Verification items for the finished model (mm, model axes). A direction names the side the tool comes from. Give positions to 0.01 mm unless a question says otherwise; leave off trailing zeros. Order: outer loops, then holes, each group sorted by start corner. A loop starts at its lowest first (then second) coordinate and runs counter-clockwise, first axis right, second up. Notation, with made-up numbers: (6, -33.75) - (57, -33.75) arc R21 cw to (57, -16.75) - close; hole circle Ø3 at (-33.5, 58.5). An arc over 180 degrees is marked (long way). Answer as a JSON object with one key per item and string values.
```python
from build123d import *

# Parameters (mm, degrees)
BOSS_EXTRUDE1_DEPTH             = 23
FILLET2_R                       = 50.8
SKETCH2_R                       = 40.05
CUT_EXTRUDE1_DEPTH              = 16
SKETCH5_R                       = 36.83
CUT_EXTRUDE2_DEPTH              = 25.4
FILLET5_R                       = 1
FILLET6_R                       = 1
CBORE_FOR_M10_SHCS7_D           = 10.5
CBORE_FOR_M10_SHCS7_CBORE_D     = 18
CBORE_FOR_M10_SHCS7_CBORE_DEPTH = 12
TAP_DRILL_FOR_M8X1_25_TAP2_D    = 6.8
F_8_0MM_DOWEL_HOLE1_D           = 8
F_8_0MM_DOWEL_HOLE1_DEPTH       = 9
F_8_0MM_DOWEL_HOLE1_TIP         = 2.403442476
F_10_0MM_DOWEL_HOLE3_D          = 10
F_10_0MM_DOWEL_HOLE3_DEPTH      = 10
F_10_0MM_DOWEL_HOLE3_TIP        = 3.004303095
CBORE_FOR_M10_SHCS9_D           = 10.5
CBORE_FOR_M10_SHCS9_CBORE_D     = 18
CBORE_FOR_M10_SHCS9_CBORE_DEPTH = 10


with BuildPart() as part:
    # Sketch1 → Boss-Extrude1 (new body)
    with BuildSketch(Plane.XY):
        with BuildLine():
            Line((84.221105008, -163.490124242), (2.699306526, -136.831626991))
            Line((2.699306526, -136.831626991), (-67.458438584, -162.730244564))
            ThreePointArc((-67.458438584, -162.730244564), (-75.680634631, -163.297391653), (-82.910842941, -159.341351783))
            Line((-82.910842941, -159.341351783), (-126.914053579, -115.336397895))
            ThreePointArc((-126.914053579, -115.336397895), (-130.093640928, -110.577690662), (-131.210211433, -104.964461595))
            Line((-131.210211433, -104.964461595), (-131.213297338, 125.035476514))
            ThreePointArc((-131.213297338, 125.035476514), (-126.350161673, 135.869915187), (-115.02264263, 139.436771249))
            Line((-115.02264263, 139.436771249), (-20.796830867, 128.37488637))
            Line((-20.796830867, 128.37488637), (49.24312976, 147.55277548))
            ThreePointArc((49.24312976, 147.55277548), (58.421803723, 147.044752766), (65.450410839, 141.119820294))
            Line((65.450410839, 141.119820294), (107.841002341, 71.642808501))
            ThreePointArc((107.841002341, 71.642808501), (117.701476238, 53.952608996), (124.683759391, 34.941564155))
            Line((124.683759391, 34.941564155), (145.845410308, -40.455794779))
            ThreePointArc((145.845410308, -40.455794779), (145.61886709, -49.11646402), (140.544799405, -56.138739339))
            Line((140.544799405, -56.138739339), (109.149264581, -79.773969292))
            Line((109.149264581, -79.773969292), (103.401152517, -150.732337669))
            ThreePointArc((103.401152517, -150.732337669), (96.90432541, -161.761540655), (84.221105008, -163.490124242))
        make_face()
    extrude(amount=BOSS_EXTRUDE1_DEPTH)

    # Fillet2
    fillet2_edges = [part.edges().sort_by_distance(p)[0] for p in [
        (109.149264581, -79.773969292, 11.5),
        (2.699306526, -136.831626991, 11.5),
        (-20.796830867, 128.37488637, 11.5),
    ]]
    fillet(fillet2_edges, radius=FILLET2_R)

    # Sketch2 → Cut-Extrude1 (cut)
    with BuildSketch(Plane(origin=(0, 0, 23), x_dir=(-1, 0, 0), z_dir=(0, 0, -1))):
        Circle(SKETCH2_R)
    extrude(amount=CUT_EXTRUDE1_DEPTH, mode=Mode.SUBTRACT)

    # Sketch5 → Cut-Extrude2 (cut)
    with BuildSketch(Plane(origin=(0, 0, 23), x_dir=(-1, 0, 0), z_dir=(0, 0, -1))):
        with Locations(Location((0, 0, 0), (0, 0, 180))):
            Circle(SKETCH5_R)
    extrude(amount=CUT_EXTRUDE2_DEPTH, mode=Mode.SUBTRACT)

    # Fillet5
    fillet5_edges = [part.edges().sort_by_distance(p)[0] for p in [
        (40.05, 0, 23),
    ]]
    fillet(fillet5_edges, radius=FILLET5_R)

    # Fillet6
    fillet6_edges = [part.edges().sort_by_distance(p)[0] for p in [
        (40.05, 0, 7),
    ]]
    fillet(fillet6_edges, radius=FILLET6_R)

    # CBORE for M10 SHCS7 (through all)
    with Locations(Plane.XY.offset(23)):
        with Locations((-116.713297339, 125.03567106), (-116.541509562, -104.964264785), (-72.538298924, -148.969218673)):
            CounterBoreHole(CBORE_FOR_M10_SHCS7_D / 2, CBORE_FOR_M10_SHCS7_CBORE_D / 2, CBORE_FOR_M10_SHCS7_CBORE_DEPTH)

    # Tap Drill for M8x1.25 Tap2 (through all)
    with Locations(Plane.XY.offset(23)):
        with Locations((46, 97.92), (-31, 98), (-105.616623552, 111.626092354), (-105.616623552, -112.292869781), (-31.12, -98.35), (45.85, -98.52), (78.925, -30.46), (77.9, 39.75)):
            Hole(TAP_DRILL_FOR_M8X1_25_TAP2_D / 2)

    # Ø8.0mm Dowel Hole1
    with Locations(Plane.XY.offset(23)):
        with Locations((-72, 97.977867106), (-72, -98.122132894)):
            Hole(F_8_0MM_DOWEL_HOLE1_D / 2, depth=F_8_0MM_DOWEL_HOLE1_DEPTH)
            with Locations((0, 0, -(F_8_0MM_DOWEL_HOLE1_DEPTH + F_8_0MM_DOWEL_HOLE1_TIP / 2))):  # 118° drill point
                Cone(0, F_8_0MM_DOWEL_HOLE1_D / 2, F_8_0MM_DOWEL_HOLE1_TIP, mode=Mode.SUBTRACT)

    # Ø10.0mm Dowel Hole3
    with Locations(Plane(origin=(0, 0, 0), x_dir=(-1, 0, 0), z_dir=(0, 0, -1))):
        with Locations((76.55340813, 103.753913834), (-59.102558089, -114.980445858)):
            Hole(F_10_0MM_DOWEL_HOLE3_D / 2, depth=F_10_0MM_DOWEL_HOLE3_DEPTH)
            with Locations((0, 0, -(F_10_0MM_DOWEL_HOLE3_DEPTH + F_10_0MM_DOWEL_HOLE3_TIP / 2))):  # 118° drill point
                Cone(0, F_10_0MM_DOWEL_HOLE3_D / 2, F_10_0MM_DOWEL_HOLE3_TIP, mode=Mode.SUBTRACT)

    # CBORE for M10 SHCS9 (through all)
    with Locations(Plane.XY.offset(23)):
        with Locations((53.072470058, 133.567563544), (131.722431635, -44.419667636), (88.780343848, -149.547952394)):
            CounterBoreHole(CBORE_FOR_M10_SHCS9_D / 2, CBORE_FOR_M10_SHCS9_CBORE_D / 2, CBORE_FOR_M10_SHCS9_CBORE_DEPTH)


solid = part.part
```
(1) Section check A-A (x = 0). Record the cut outline in (y, z), then the cut area to 3 significant figures.
Computed values:
{"outline": "(-139.94, 0) - (-36.83, 0) - (-36.83, 7) - (-39.05, 7) arc R1 cw to (-40.05, 8) - (-40.05, 22) arc R1 ccw to (-41.05, 23) - (-139.94, 23) - close; (36.83, 0) - (134.07, 0) - (134.07, 23) - (41.05, 23) arc R1 ccw to (40.05, 22) - (40.05, 8) arc R1 cw to (39.05, 7) - (36.83, 7) - close", "area": "4,510 mm²"}
(2) Gauge pin test, flat ends, axial feed: pin 1 Ø9 at (x, y) = (53.5, 133.5) entering from +Z; pin 2 Ø13.5 at (x, y) = (-116.54, -104.96) entering from +Z; pin 3 Ø12 at (x, z) = (72.5, 7) entering from +Y; pin 4 Ø8 at (x, z) = (40, 16.5) entering from +Y. Record the tip position at first contact, or that the pin passes through.
Computed values:
{"pin 1": "passes through", "pin 2": "stops at z = 11", "pin 3": "stops at y = 139.4", "pin 4": "stops at y = 146.12"}
(3) Material ranges on line 1 along X through (y, z) = (-98, 8.5); line 2 along Y through (x, z) = (-33, 11.75); line 3 along Y through (x, z) = (-72, 19.5), recorded low to high. Write a range as [from, to].
Computed values:
{"line 1": "x = [-131.21, -34.5], [-27.74, 42.49], [49.21, 107.88]", "line 2": "y = [-150.01, -101.18], [-95.52, -22.69], [22.69, 95.25], [100.75, 129.81]", "line 3": "y = [-163.63, -157.95], [-139.99, -102.12], [-94.12, 93.98], [101.98, 134.39]"}
(4) Section check B-B (y = 0). Record the cut outline in (x, z), then the cut area to 3 significant figures.
Computed values:
{"outline": "(-131.21, 0) - (-36.83, 0) - (-36.83, 7) - (-39.05, 7) arc R1 cw to (-40.05, 8) - (-40.05, 22) arc R1 ccw to (-41.05, 23) - (-131.21, 23) - close; (36.83, 0) - (134.49, 0) - (134.49, 23) - (41.05, 23) arc R1 ccw to (40.05, 22) - (40.05, 8) arc R1 cw to (39.05, 7) - (36.83, 7) - close", "area": "4,310 mm²"}
(5) Section check D-D (y = -129.5). Record the cut outline in (x, z).
Computed values:
{"outline": "(-112.75, 0) - (105.12, 0) - (105.12, 23) - (-112.75, 23) - close"}
(6) Access from +Z, -Z, +X, -X, +Y, -Y to the whole of each face (thin tool, end or side, straight path). Record for faces 5 (the flat face through (-40.295, -152.703, 11.339)), 6 (the flat face through (105.38, -126.29, 11.34)), 7 (the flat face through (-112.7, -108.8, 11)).
Computed values:
{"face 5": "+Z, -Z, -Y", "face 6": "+Z, -Z, +X, -Y", "face 7": "+Z"}
(7) Section check C-C (z = 3.5). Count the separate pieces of the cut face and the enclosed holes in it, then the cut area to 3 significant figures.
Computed values:
{"separate pieces": "1", "enclosed holes": "17", "area": "65,100 mm²"}
(8) Release check for a two-part mould opening along X. For faces 1 (the cylindrical face through (97.058, -161.658, 11.339)), 2 (the cylindrical face through (82.32, -30.31, 11.34)), 3 (the flat face through (-21, -41, 0)), 4 (the cylindrical face through (-123.175, -98.882, 17.084)) record: pulls with the +X half, pulls with the -X half, needs draft (parallel to the pull), parting line crosses it, or undercut.
Computed values:
{"face 1": "parting line crosses it", "face 2": "undercut", "face 3": "needs draft", "face 4": "undercut"}
